Input: part model. Units: mm. Frame: model coordinates. Face numbers are marked on the shaded views. Give positions to 0.01 mm unless a question says otherwise; leave off trailing zeros. Order: outer loops, then holes, each group sorted by start corner. A loop starts at its lowest first (then second) coordinate and runs counter-clockwise, first axis right, second up. Notation, with made-up numbers: (21, 16) -> (54, 16) arc R17 cw to (54, 21) -> close; hole circle Ø2 at (7, -32.75). An arc over 180 degrees is marked (long way). Use a Markdown table: item, result. Add a question column.
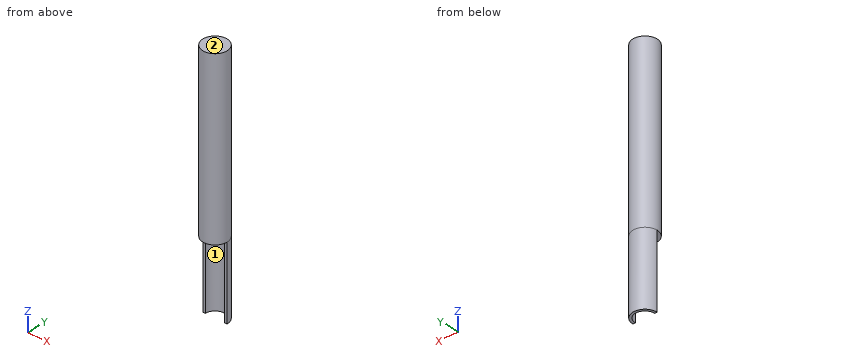
from build123d import *

# Parameters (mm, degrees)
F0_R     = 0.5
F1_DEPTH = 7
F3_DEPTH = 3


with BuildPart() as f1:
    # F0 (on Top) → F1 (new body)
    with BuildSketch(Plane.XY):
        Circle(F0_R)
    extrude(amount=F1_DEPTH)

    # F2 (on face) → F3 (join)
    with BuildSketch(Plane(origin=(0, 0, 0), x_dir=(1, 0, 0), z_dir=(0, 0, -1))):
        with BuildLine():
            Line((-0.4, 0), (-0.5, 0))
            ThreePointArc((-0.5, 0), (0, -0.5), (0.5, 0))
            Line((0.5, 0), (0.4, 0))
            ThreePointArc((0.4, 0), (0, -0.4), (-0.4, 0))
        make_face()
    extrude(amount=F3_DEPTH)


solid = f1.part
Q1. Section query C-C (z = 1.25). Return loops of the section in (x, y).
Q2. Section query B-B (y = 0.2). Return loops of the section in (x, z), plus the area to 3 significant figures.
Q3. Ray query, line 1 (Z direction, x = 0.2, y = -0.1); line 2 (X direction, y = 0.05, z = 2); line 3 (X direction, y = 0.3, z = 0.5). Return the intervals inside material, ascending.
Q4. First-contact query: pin 1 (0.5 mm diameter, centred on x = 0, y = -0.5, fed in from -Z). Flat tip, straight axial feed; report the tip coordinate or a pass-through.
Q5. Draft query along X for the marked faces 1 and 2. Return one class per face: +X half, -X half, draft (parallel to the pull), parting line (faces both ways), or undercut.
Q6. Section query A-A (x = 0). Return loops of the section in (y, z), plus the area to 3 significant figures.
Solution:
| question | item | result |
|---|---|---|
| 1 | outline | circle Ø1 at (0, 0) |
| 2 | outline | (-0.46, -3) -> (-0.35, -3) -> (-0.35, 0) -> (0.35, 0) -> (0.35, -3) -> (0.46, -3) -> (0.46, 7) -> (-0.46, 7) -> close |
| 2 | area | 7.09 mm² |
| 3 | line 1 | z = 0 to 7 |
| 3 | line 2 | x = -0.5 to 0.5 |
| 3 | line 3 | x = -0.4 to 0.4 |
| 4 | pin 1 | stops at z = 0 |
| 5 | face 1 | undercut |
| 5 | face 2 | draft |
| 6 | outline | (-0.5, 0) -> (0.4, 0) -> (0.4, -3) -> (0.5, -3) -> (0.5, 7) -> (-0.5, 7) -> close |
| 6 | area | 7.30 mm² |
